Geometry: final body of the model. Coordinates: model frame, mm. Face numbers are marked on the shaded views. A direction names the side the tool comes from. Give positions to 0.01 mm unless a question says otherwise; leave off trailing zeros. Write each loop counter-clockwise with the first axis right and the second up, starting at its lowest first coordinate (ties: lowest second). Pieces come first, ordered by that corner, then holes.
Q1. Line query: L1, parallel to X at y = 52, z = 17 (3 decimals); L2, parallel to Y at x = 62, z = 41.5; L3, parallel to X at y = -39.5, z = -8 (3 decimals). Output: solid intervals per line, ascending.
Q2. Reachability of the marked faces 1, 2 and 3 from +Z, -Z, +X, -X, +Y, -Y: full face, straight path, thin tool, end or side. Return the list, or none.
Q3. Cut plane D-D on x = 29. Return the cut outline in (y, z), plus the area to 3 significant figures.
Q4. Cut plane B-B on x = 58. Count the separate pieces of the cut face and the enclosed holes in it, plus the area to 3 significant figures.
Q5. Pin query (flat end, axial travel): pin 1 (8 mm diameter, centred on y = 57, z = 22.5, fed in from -X); pin 2 (8 mm diameter, centred on x = 59, z = 32.5, fed in from -Y); pin 3 (8 mm diameter, centred on x = 23.5, z = -11, fed in from -Y). Return the tip coordinate at first contact, or that it passes through.
Q6. Cut plane A-A on x = 43.5. Return the cut outline in (y, z), plus the area to 3 significant figures.
Q7. Draft query along X for the marked faces 4, 5, 6 and 7. Return one class per face: pulls with the +X half, pulls with the -X half, needs draft (parallel to the pull), parting line crosses it, or undercut.
```python
from build123d import *

# Parameters (mm, degrees)
SALIENTE_EXTRUIR1_START = 16.51
CROQUIS2_R              = 6.731
CROQUIS2_R_2            = 25.4
SALIENTE_EXTRUIR1_DEPTH = 16.51
CORTAR_EXTRUIR1_REACH   = 129.898
CROQUIS3_R              = 9.525
CHAFL_N1_SIZE           = 0.8128
CHAFL_N2_SIZE           = 3.175
REDONDEO1_R             = 1.524
CROQUIS4_R              = 25.4
CROQUIS4_R_2            = 6.731
SALIENTE_EXTRUIR2_DEPTH = 16.51
CROQUIS6_R              = 76.2
CROQUIS6_R_2            = 9.525
CROQUIS6_R_3            = 25.4
SALIENTE_EXTRUIR3_DEPTH = 16.51


with BuildPart() as part:
    # Croquis1 → Revolución1 (revolve)
    with BuildSketch(Plane.XY, mode=Mode.PRIVATE) as revoluci_n1_sk:
        Polygon((0, 25.4), (53.975, 25.4), (53.975, 47.625), (52.3748, 46.0248), (52.3748, 34.29), (34.925, 34.29), (16.51, 38.204229083), (16.51, 76.2), (1.6002, 76.2), (1.6002, 47.6377), (0, 46.0375), align=None)
    revolve(revoluci_n1_sk.sketch.rotate(Axis((0, 0, 0), (1, 0, 0)), 90), axis=Axis((0, 0, 0), (1, 0, 0)))

    # Croquis2 → Saliente-Extruir1 (add)
    with BuildSketch(Plane(origin=(53.975, 0, 0), x_dir=(0, 0, -1), z_dir=(1, 0, 0)).offset(SALIENTE_EXTRUIR1_START)):
        with BuildLine():
            Line((-60.071, 40.132), (-60.071, 24.4523651))
            ThreePointArc((-60.071, 24.4523651), (-60.317121003, 20.92499052), (-61.050714286, 17.465975072))
            ThreePointArc((-61.050714286, 17.465975072), (-63.5, 0), (-61.050714286, -17.465975072))
            ThreePointArc((-61.050714286, -17.465975072), (-60.317121003, -20.92499052), (-60.071, -24.4523651))
            Line((-60.071, -24.4523651), (-60.071, -40.132))
            ThreePointArc((-60.071, -40.132), (-54.23100211, -54.23100211), (-40.132, -60.071))
            Line((-40.132, -60.071), (-24.4523651, -60.071))
            ThreePointArc((-24.4523651, -60.071), (-20.92499052, -60.317121003), (-17.465975072, -61.050714286))
            ThreePointArc((-17.465975072, -61.050714286), (0, -63.5), (17.465975072, -61.050714286))
            ThreePointArc((17.465975072, -61.050714286), (20.92499052, -60.317121003), (24.4523651, -60.071))
            Line((24.4523651, -60.071), (40.132, -60.071))
            ThreePointArc((40.132, -60.071), (54.23100211, -54.23100211), (60.071, -40.132))
            Line((60.071, -40.132), (60.071, -24.4523651))
            ThreePointArc((60.071, -24.4523651), (60.317121003, -20.92499052), (61.050714286, -17.465975072))
            ThreePointArc((61.050714286, -17.465975072), (63.5, 0), (61.050714286, 17.465975072))
            ThreePointArc((61.050714286, 17.465975072), (60.317121003, 20.92499052), (60.071, 24.4523651))
            Line((60.071, 24.4523651), (60.071, 40.132))
            ThreePointArc((60.071, 40.132), (54.23100211, 54.23100211), (40.132, 60.071))
            Line((40.132, 60.071), (24.4523651, 60.071))
            ThreePointArc((24.4523651, 60.071), (20.92499052, 60.317121003), (17.465975072, 61.050714286))
            ThreePointArc((17.465975072, 61.050714286), (0, 63.5), (-17.465975072, 61.050714286))
            ThreePointArc((-17.465975072, 61.050714286), (-20.92499052, 60.317121003), (-24.4523651, 60.071))
            Line((-24.4523651, 60.071), (-40.132, 60.071))
            ThreePointArc((-40.132, 60.071), (-54.23100211, 54.23100211), (-60.071, 40.132))
        make_face()
        with Locations((-42.656216575, 42.656216575)):
            Circle(CROQUIS2_R, mode=Mode.SUBTRACT)
        with Locations((42.656216575, 42.656216575)):
            Circle(CROQUIS2_R, mode=Mode.SUBTRACT)
        with Locations((42.656216575, -42.656216575)):
            Circle(CROQUIS2_R, mode=Mode.SUBTRACT)
        with Locations((-42.656216575, -42.656216575)):
            Circle(CROQUIS2_R, mode=Mode.SUBTRACT)
        with Locations(Location((0, 0, 0), (0, 0, 180))):
            Circle(CROQUIS2_R_2, mode=Mode.SUBTRACT)
    extrude(amount=-SALIENTE_EXTRUIR1_DEPTH)

    # Croquis3 → Cortar-Extruir1 (cut, up to next)
    with BuildSketch(Plane.ZY.offset(-1.6002), mode=Mode.PRIVATE) as cortar_extruir1_sk1:
        with Locations((-42.656216575, 42.656216575)):
            Circle(CROQUIS3_R)
    cortar_extruir1_tool1 = extrude(cortar_extruir1_sk1.sketch, amount=-CORTAR_EXTRUIR1_REACH, mode=Mode.PRIVATE) & part.part
    # Croquis3 → Cortar-Extruir1 (cut, up to next)
    with BuildSketch(Plane.ZY.offset(-1.6002), mode=Mode.PRIVATE) as cortar_extruir1_sk2:
        with Locations((42.656216575, 42.656216575)):
            Circle(CROQUIS3_R)
    cortar_extruir1_tool2 = extrude(cortar_extruir1_sk2.sketch, amount=-CORTAR_EXTRUIR1_REACH, mode=Mode.PRIVATE) & part.part
    # Croquis3 → Cortar-Extruir1 (cut, up to next)
    with BuildSketch(Plane.ZY.offset(-1.6002), mode=Mode.PRIVATE) as cortar_extruir1_sk3:
        with Locations((42.656216575, -42.656216575)):
            Circle(CROQUIS3_R)
    cortar_extruir1_tool3 = extrude(cortar_extruir1_sk3.sketch, amount=-CORTAR_EXTRUIR1_REACH, mode=Mode.PRIVATE) & part.part
    # Croquis3 → Cortar-Extruir1 (cut, up to next)
    with BuildSketch(Plane.ZY.offset(-1.6002), mode=Mode.PRIVATE) as cortar_extruir1_sk4:
        with Locations((-42.656216575, -42.656216575)):
            Circle(CROQUIS3_R)
    cortar_extruir1_tool4 = extrude(cortar_extruir1_sk4.sketch, amount=-CORTAR_EXTRUIR1_REACH, mode=Mode.PRIVATE) & part.part
    add(cortar_extruir1_tool1.solids().sort_by_distance((1.6002, 42.656217, -42.656217))[0], mode=Mode.SUBTRACT)
    add(cortar_extruir1_tool2.solids().sort_by_distance((1.6002, 42.656217, 42.656217))[0], mode=Mode.SUBTRACT)
    add(cortar_extruir1_tool3.solids().sort_by_distance((1.6002, -42.656217, 42.656217))[0], mode=Mode.SUBTRACT)
    add(cortar_extruir1_tool4.solids().sort_by_distance((1.6002, -42.656217, -42.656217))[0], mode=Mode.SUBTRACT)

    # Chaflán1
    chafl_n1_edges = [part.edges().sort_by_distance(p)[0] for p in [
        (53.975, 42.656216575, 49.387216575),
        (53.975, 42.656216575, -35.925216575),
        (53.975, -42.656216575, -35.925216575),
        (53.975, -42.656216575, 49.387216575),
        (70.485, 42.656216575, 49.387216575),
        (70.485, 42.656216575, -35.925216575),
        (70.485, -42.656216575, -35.925216575),
        (70.485, -42.656216575, 49.387216575),
        (1.6002, 0, -76.2),
        (16.51, 0, -76.2),
        (1.6002, -42.656216575, -52.181216575),
        (16.51, -42.656216575, -52.181216575),
        (1.6002, -42.656216575, 33.131216575),
        (16.51, -42.656216575, 33.131216575),
        (1.6002, 42.656216575, 33.131216575),
        (16.51, 42.656216575, 33.131216575),
        (1.6002, 42.656216575, -52.181216575),
        (16.51, 42.656216575, -52.181216575),
    ]]
    chamfer(chafl_n1_edges, length=CHAFL_N1_SIZE)

    # Chaflán2
    chafl_n2_edges = [part.edges().sort_by_distance(p)[0] for p in [
        (0, 0, -25.4),
        (70.485, 0, -25.4),
    ]]
    chamfer(chafl_n2_edges, length=CHAFL_N2_SIZE)

    # Redondeo1
    redondeo1_edges = [part.edges().sort_by_distance(p)[0] for p in [
        (52.3748, 0, -34.29),
        (16.51, 0, -38.204229083),
    ]]
    fillet(redondeo1_edges, radius=REDONDEO1_R)


with BuildPart() as body_2:
    # Croquis4 → Saliente-Extruir2 (new body)
    with BuildSketch(Plane(origin=(70.485, 0, 0), x_dir=(0, 0, -1), z_dir=(1, 0, 0))):
        with BuildLine():
            Line((-24.4523651, 60.071), (-40.132, 60.071))
            ThreePointArc((-40.132, 60.071), (-54.23100211, 54.23100211), (-60.071, 40.132))
            Line((-60.071, 40.132), (-60.071, 24.4523651))
            ThreePointArc((-60.071, 24.4523651), (-60.317121003, 20.92499052), (-61.050714286, 17.465975072))
            ThreePointArc((-61.050714286, 17.465975072), (-63.5, 0), (-61.050714286, -17.465975072))
            ThreePointArc((-61.050714286, -17.465975072), (-60.317121003, -20.92499052), (-60.071, -24.4523651))
            Line((-60.071, -24.4523651), (-60.071, -40.132))
            ThreePointArc((-60.071, -40.132), (-54.23100211, -54.23100211), (-40.132, -60.071))
            Line((-40.132, -60.071), (-24.4523651, -60.071))
            ThreePointArc((-24.4523651, -60.071), (-20.92499052, -60.317121003), (-17.465975072, -61.050714286))
            ThreePointArc((-17.465975072, -61.050714286), (0, -63.5), (17.465975072, -61.050714286))
            ThreePointArc((17.465975072, -61.050714286), (20.92499052, -60.317121003), (24.4523651, -60.071))
            Line((24.4523651, -60.071), (40.132, -60.071))
            ThreePointArc((40.132, -60.071), (54.23100211, -54.23100211), (60.071, -40.132))
            Line((60.071, -40.132), (60.071, -24.4523651))
            ThreePointArc((60.071, -24.4523651), (60.317121003, -20.92499052), (61.050714286, -17.465975072))
            ThreePointArc((61.050714286, -17.465975072), (63.5, 0), (61.050714286, 17.465975072))
            ThreePointArc((61.050714286, 17.465975072), (60.317121003, 20.92499052), (60.071, 24.4523651))
            Line((60.071, 24.4523651), (60.071, 40.132))
            ThreePointArc((60.071, 40.132), (54.23100211, 54.23100211), (40.132, 60.071))
            Line((40.132, 60.071), (24.4523651, 60.071))
            ThreePointArc((24.4523651, 60.071), (20.92499052, 60.317121003), (17.465975072, 61.050714286))
            ThreePointArc((17.465975072, 61.050714286), (0, 63.5), (-17.465975072, 61.050714286))
            ThreePointArc((-17.465975072, 61.050714286), (-20.92499052, 60.317121003), (-24.4523651, 60.071))
        make_face()
        Circle(CROQUIS4_R, mode=Mode.SUBTRACT)
        with Locations((42.656216575, -42.656216575)):
            Circle(CROQUIS4_R_2, mode=Mode.SUBTRACT)
        with Locations((-42.656216575, -42.656216575)):
            Circle(CROQUIS4_R_2, mode=Mode.SUBTRACT)
        with Locations((42.656216575, 42.656216575)):
            Circle(CROQUIS4_R_2, mode=Mode.SUBTRACT)
        with Locations((-42.656216575, 42.656216575)):
            Circle(CROQUIS4_R_2, mode=Mode.SUBTRACT)
    extrude(amount=SALIENTE_EXTRUIR2_DEPTH)


with BuildPart() as body_3:
    # Croquis5 → Revolución2 (revolve)
    with BuildSketch(Plane.XY, mode=Mode.PRIVATE) as revoluci_n2_sk:
        with BuildLine():
            Line((86.995, -25.4), (156.845, -25.4))
            Line((156.845, -25.4), (156.845, -38.1))
            Line((156.845, -38.1), (141.097, -38.1))
            Line((141.097, -38.1), (100.143007491, -49.07358922))
            ThreePointArc((100.143007491, -49.07358922), (93.625730565, -50.369956202), (86.995, -50.804557244))
            Line((86.995, -50.804557244), (86.995, -25.4))
        make_face()
    revolve(revoluci_n2_sk.sketch.rotate(Axis((0, 0, 0), (1, 0, 0)), 90), axis=Axis((0, 0, 0), (1, 0, 0)))


with BuildPart() as body_4:
    # Croquis6 → Saliente-Extruir3 (new body)
    with BuildSketch(Plane(origin=(156.845, 0, 0), x_dir=(0, 0, -1), z_dir=(1, 0, 0))):
        with Locations(Location((0, 0, 0), (0, 0, 180))):
            Circle(CROQUIS6_R)
        with Locations(Location((42.656216575, -42.656216575, 0), (0, 0, 180))):
            Circle(CROQUIS6_R_2, mode=Mode.SUBTRACT)
        with Locations(Location((-42.656216575, -42.656216575, 0), (0, 0, 180))):
            Circle(CROQUIS6_R_2, mode=Mode.SUBTRACT)
        with Locations(Location((42.656216575, 42.656216575, 0), (0, 0, 180))):
            Circle(CROQUIS6_R_2, mode=Mode.SUBTRACT)
        with Locations(Location((-42.656216575, 42.656216575, 0), (0, 0, 180))):
            Circle(CROQUIS6_R_2, mode=Mode.SUBTRACT)
        Circle(CROQUIS6_R_3, mode=Mode.SUBTRACT)
    extrude(amount=SALIENTE_EXTRUIR3_DEPTH)


solid = part.part
```
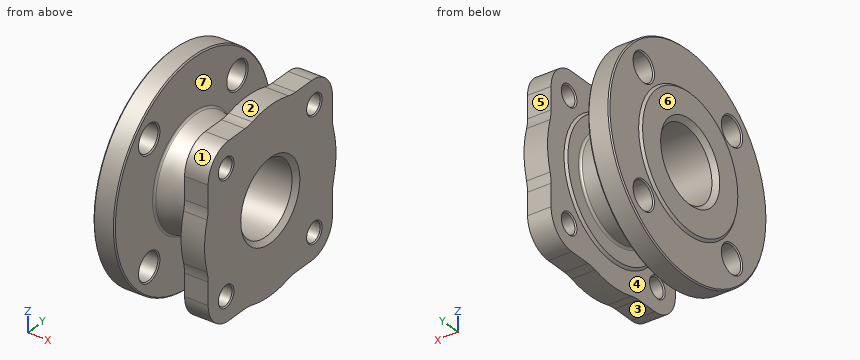
Data:
1. L1: x = 1.6 to 16.51, 53.975 to 70.485
1. L2: y = -60.02 to -49.29, -36.03 to 36.03, 49.29 to 60.02
1. L3: x = 0 to 16.51, 52.375 to 70.485
2. face 1: +Z, +X, -Y
2. face 2: +Z, +X
2. face 3: -Z, +X, -Y
3. outline: circle Ø71.1 at (0, 0); hole circle Ø50.8 at (0, 0)
3. area: 1,940 mm2
4. separate pieces: 1
4. enclosed holes: 5
4. area: 11,900 mm2
5. pin 1: stops at x = 1.6
5. pin 2: stops at y = -60.07
5. pin 3: stops at y = -36.41
6. outline: circle Ø68.58 at (0, 0); hole circle Ø50.8 at (0, 0)
6. area: 1,670 mm2
7. face 4: undercut
7. face 5: needs draft
7. face 6: pulls with the -X half
7. face 7: undercut
